from build123d import *

# Parameters (mm, degrees)
F1_DEPTH = 63.5
F0_W     = 25.4
F0_H     = 19.05
F2_DEPTH = 50.8
F3_DEPTH = 7.9375
F5_R     = 6.35
F6_R     = 6.35


with BuildPart() as f1:
    # F0 (on Front) → F1 (new body, symmetric)
    with BuildSketch(Plane.XZ):
        Polygon((-41.275, 9.525), (-41.275, -9.525), (41.275, -9.525), (41.275, 9.525), (22.225, 9.525), align=None)
    extrude(amount=F1_DEPTH, both=True)

    # F0 (on Front) → F2 (join)
    with BuildSketch(Plane.XZ):
        with Locations((73.025, 52.4002)):
            Rectangle(F0_W, F0_H)
        with BuildLine():
            Line((22.225, 9.525), (41.275, 9.525))
            Line((41.275, 9.525), (41.275, 27.0002))
            ThreePointArc((41.275, 27.0002), (45.9246798487, 38.2255201513), (57.15, 42.8752))
            Line((57.15, 42.8752), (60.325, 42.8752))
            Line((60.325, 42.8752), (60.325, 61.9252))
            Line((60.325, 61.9252), (57.15, 61.9252))
            add(Edge.make_bspline(
                [(56.6563688667, 61.9217113262), (56.8210697668, 61.9232432232), (56.985614657, 61.924406559), (57.15, 61.9252)],
                knots=[111.0767656068, 111.0767656068, 111.0767656068, 111.0767656068, 111.5045361635, 111.5045361635, 111.5045361635, 111.5045361635], degree=3))
            ThreePointArc((56.6563688667, 61.9217113262), (32.2803830716, 51.5207582896), (22.225, 27.0002))
            Line((22.225, 27.0002), (22.225, 9.525))
        make_face()
    extrude(amount=F2_DEPTH)

    # F0 (on Front) → F3 (join, symmetric)
    with BuildSketch(Plane.XZ):
        with BuildLine():
            add(Edge.make_bspline(
                [(-41.275, 9.525), (-39.3966058036, 36.2756986169), (13.8894158841, 61.52393227), (56.6563688667, 61.9217113262)],
                knots=[0, 0, 0, 0, 111.0767656068, 111.0767656068, 111.0767656068, 111.0767656068], degree=3))
            Line((-41.275, 9.525), (22.225, 9.525))
            Line((22.225, 9.525), (22.225, 27.0002))
            ThreePointArc((22.225, 27.0002), (32.2803830716, 51.5207582896), (56.6563688667, 61.9217113262))
        make_face()
    extrude(amount=F3_DEPTH, both=True)

    # F0 (on Front) → F4 (revolve)
    with BuildSketch(Plane.XZ):
        Polygon((85.725, 66.675), (85.725, 61.9252), (85.725, 42.8752), (85.725, 38.1), (111.125, 38.1), (111.125, 66.675), align=None)
    revolve(axis=Axis((85.725, 0, 54.7751), (0, 0, 1)))

    # F5
    f5_edges = [f1.edges().sort_by_distance(p)[0] for p in [
        (-41.275, -63.5, 0),
        (41.275, -63.5, 0),
        (41.275, 63.5, 0),
    ]]
    fillet(f5_edges, radius=F5_R)

    # F6
    f6_edges = [f1.edges().sort_by_distance(p)[0] for p in [
        (-41.275, 63.5, 0),
    ]]
    fillet(f6_edges, radius=F6_R)


solid = f1.part
Work out the finished part from the listing and answer in its coordinate system (mm). A direction names the side the tool comes from. Give positions to 0.01 mm unless a question says otherwise; leave off trailing zeros. Order: outer loops, then holes, each group sorted by start corner. A loop starts at its lowest first (then second) coordinate and runs counter-clockwise, first axis right, second up. Notation, with made-up numbers: (71, 29) -> (76, 29) arc R12 ccw to (76, 44) -> close; hole circle Ø1 at (82.5, 46.5). An arc over 180 degrees is marked (long way). One line per item, written item: value.
Item 1: Determine the mould class of faces 4 (the flat face through (68, -31, 42.875)), 5 (the flat face through (-3, -7.938, 30)), 6 (the flat face through (-41.275, -1, 0)), 7 (the cylindrical face through (32.015, 3.913, 51.248)) for opening direction X: released by +X, released by -X, zero draft, split by the parting line, or undercut.
Answer sheet:
face 4: undercut
face 5: zero draft
face 6: released by -X
face 7: undercut
Item 2: Find section A-A, the plane z = 0.5. Give the vertices of the cut face in (x, y) (3 decimals), plus the area to 3 significant figures.
Answer sheet:
outline: (-41.275, -57.15) arc R6.35 ccw to (-34.925, -63.5) -> (34.925, -63.5) arc R6.35 ccw to (41.275, -57.15) -> (41.275, 57.15) arc R6.35 ccw to (34.925, 63.5) -> (-34.925, 63.5) arc R6.35 ccw to (-41.275, 57.15) -> close
area: 10,400 mm²
Item 3: Flat-ended cylindrical pins translate along their axes: P1, Ø1, axis at x = -4.5, y = 6.5, coming from the +Z side; P2, Ø12, axis at y = -41, z = 16.5, coming from the -X side (3 decimals); P3, Ø15.5, axis at x = 4.5, z = 25.5, coming from the +Y side. Find the tip coordinate at first contact, or state that the pin passes through.
Answer sheet:
P1: z = 47.41
P2: x = 22.225
P3: y = 7.94
Item 4: Straight lines are drawn through the part: probe 1 along Y at (x, z) = (23, 13); probe 2 along Z at (x, y) = (9, 58) (3 decimals); probe 3 along X at (y, z) = (-18, 22.5) (3 decimals). For each, find the intervals that lie inside material, in ascending order.
Answer sheet:
probe 1: -50.8 to 0
probe 2: -9.525 to 9.525
probe 3: 22.225 to 41.275
Item 5: A tool of negligible diameter and unlimited length cuts with its end or side. For faces 1 (the flat face through (46, -50.8, 42)), 2 (the flat face through (37, 0, 36)), 3 (the flat face through (85.725, -38, 52)), from which of +Z, -Z, +X, -X, +Y, -Y can it reach the whole face along a straight path? Write none if from no direction.
Answer sheet:
face 1: +Z, +X, -X, -Y
face 2: +Y
face 3: +Z, -Z, +X, -Y
Item 6: Find section B-B, the plane y = 20. Give the vertices of the cut face in (x, z) (3 decimals).
Answer sheet:
outline: (-41.275, -9.525) -> (41.275, -9.525) -> (41.275, 9.525) -> (-41.275, 9.525) -> close; (70.067, 38.1) -> (101.383, 38.1) -> (101.383, 66.675) -> (70.067, 66.675) -> close
